Study the drawing (mm; zero at the part's minimum x, y, z) and answer. Give positions to 0.01 mm unless a question says otherwise; leave off trailing zeros. Loops run counter-clockwise (first coordinate to the right, second up) from the corner with the lowest first, then second, coordinate; pieces in that order, holes last. Notation, with made-up numbers: M 86.25,44.5 L 123.25,44.5 A13 ccw 123.25,49.5 Z; hole C 38.25,-8 d4. An arc over 180 degrees is marked long. Use one line per item in the form item = value. Start each with the question number.
1. The part is cut by section B-B (x = 25). Write down the section's boundary in (y, z) (1 decimal).
2. The part is cut by section C-C (y = 28.5). Write down the section's boundary in (x, z) (1 decimal), and give its area (3 significant figures).
3. Each of these flat-tipped pins is pushed along its axis until it touches: pin 1 Ø1 at (y, z) = (16, 44.5) entering from -X; pin 2 Ø15 at (x, z) = (32.92, 29.1) entering from -Y. Where does it stop, or does it pass through?
4. Straight lines are drawn through the part: line 1 (X direction, y = 3.5, z = 26.5) (1 decimal); line 2 (X direction, y = 43.5, z = 33); line 3 (Z direction, x = 37, y = 36.5). For each, find the intervals that lie inside material, in ascending order. Write a range as from..to.
5. The part is cut by section A-A (z = 38.5). Write down the section's boundary in (x, y) (1 decimal).
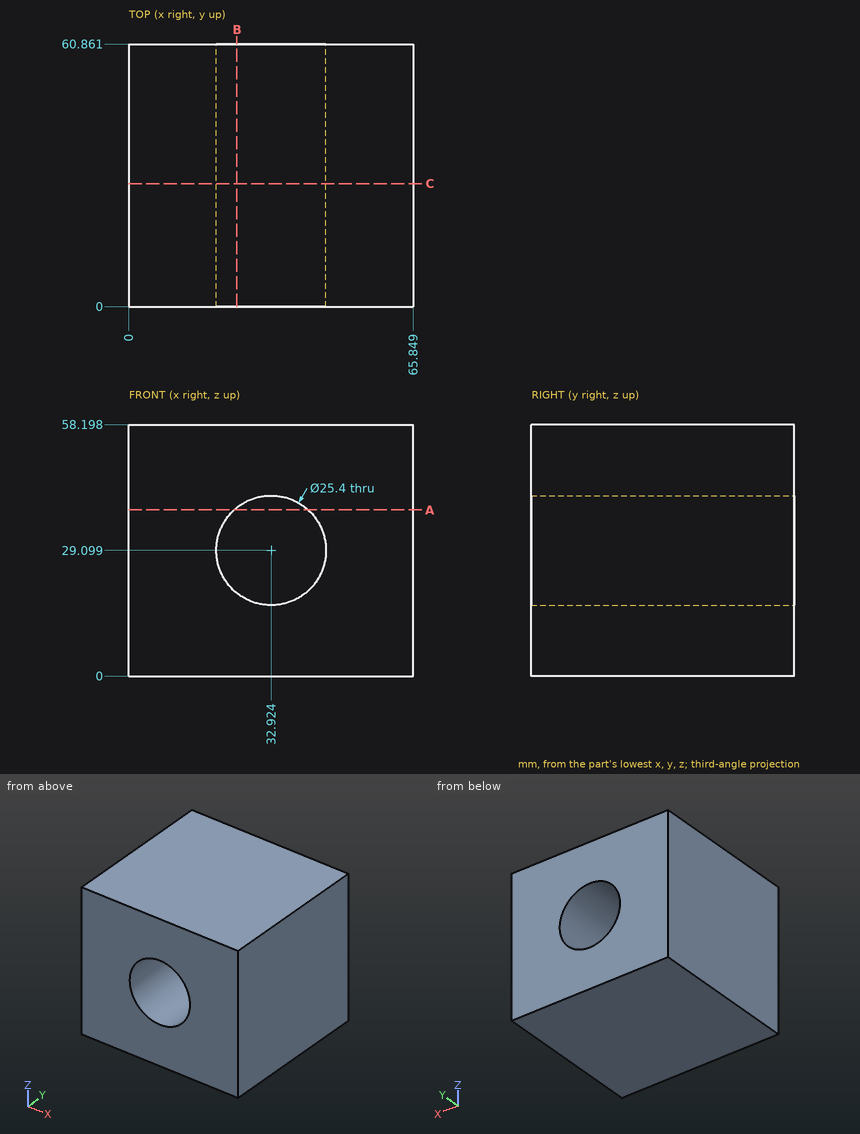
Derived:
q1.outline = M 0,0 L 60.9,0 L 60.9,19.2 L 0,19.2 Z; M 0,39 L 60.9,39 L 60.9,58.2 L 0,58.2 Z
q2.outline = M 0,0 L 65.8,0 L 65.8,58.2 L 0,58.2 Z; hole C 32.9,29.1 d25.4
q2.area = 3,330 mm2
q3.pin_1 = 0
q3.pin_2 = through
q4.line_1 = 0..20.5, 45.4..65.8
q4.line_2 = 0..20.84, 45.01..65.85
q4.line_3 = 0..17.07, 41.13..58.2
q5.outline = M 0,0 L 24.4,0 L 24.4,60.9 L 0,60.9 Z; M 41.5,0 L 65.8,0 L 65.8,60.9 L 41.5,60.9 Z
